from build123d import *

# Parameters (mm, degrees)
EXTRUDE_1_DEPTH     = 0.6
SKETCH_2_W          = 6
SKETCH_2_H          = 0.6
EXTRUDE_2_DEPTH     = 2.5
SKETCH_3_W          = 6
SKETCH_3_H          = 1.9
CUT_EXTRUDE_1_DEPTH = 42.859885332


with BuildPart() as part:
    # 草图1 → 凸台-拉伸1 (new body)
    with BuildSketch(Plane.XY):
        Polygon((0, 0), (11.5, 0), (11.5, 3), (18, 3), (18, 0), (39, 0), (39, 6.8), (33.2, 6.8), (31, 9), (16, 9), (16, 15), (10, 15), (10, 12.5), (0, 12.5), (0, 9), (10, 9), (10, 6.5), (0, 6.5), align=None)
    extrude(amount=EXTRUDE_1_DEPTH)

    # 草图2 → 凸台-拉伸2 (add)
    with BuildSketch(Plane(origin=(0, 0, 0), x_dir=(-1, 0, 0), z_dir=(0, 0, -1))):
        with Locations((-13, 12.8)):
            Rectangle(SKETCH_2_W, SKETCH_2_H)
    extrude(amount=EXTRUDE_2_DEPTH)

    # 草图3 → 切除-拉伸1 (cut, through all)
    with BuildSketch(Plane(origin=(0, 0, 0), x_dir=(-1, 0, 0), z_dir=(0, 0, -1))):
        with Locations((-13, 14.05)):
            Rectangle(SKETCH_3_W, SKETCH_3_H)
    extrude(amount=-CUT_EXTRUDE_1_DEPTH, mode=Mode.SUBTRACT)


solid = part.part
The model under review builds one solid part; all positions refer to its coordinate system, in mm. A direction names the side the tool comes from. Round coordinates to 2 decimals unless told otherwise and drop trailing zeros. Write each loop counter-clockwise with the first axis right and the second up, starting at its lowest first coordinate (ties: lowest second). Pieces come first, ordered by that corner, then holes. Notation, with made-up numbers: M -15.5,-32 L -6.5,-32 A27 cw -6.5,-15 Z; hole C 44.5,-16 d11. An arc over 180 degrees is marked long. Use a Markdown table: item, result. Add a question column.
Q1. To check wall thickness, follow line 1 (Y direction, x = 5, z = 0.25); line 2 (Z direction, x = 4, y = 3.25); line 3 (Y direction, x = 12, z = 0.4). State the ranges of each line that lie inside material, in increasing order.
Q2. We need section C-C, the plane z = -1.4. State the section outline as (x, y) points.
Q3. We need section A-A, the plane x = 15. State the section outline as (y, z) points, plus the area to 3 significant figures.
Q4. Machinability: for faces 1 (the face through (13, 12.5, -1)), 2 (the face through (13, 13.1, -1)), 3 (the face through (16, 11.6, 0.3)), which of the approach directions +Z, -Z, +X, -X, +Y, -Y give a long, thin tool a straight path to every point of the face, cutting with its end or side? Answer none if there is none.
Q5. Insertion check: pin 1 (1.2 mm diameter, centred on x = 11.5, z = -1, fed in from -Y); pin 2 (6 mm diameter, centred on x = 17, y = 4, fed in from -Z); pin 3 (1.5 mm diameter, centred on x = 4.5, y = 8, fed in from +Z); pin 4 (0.5 mm diameter, centred on x = 7, z = 0.5, fed in from +Y). Each pin has a flat end and moves straight along its axis. Give the tip position at first contact, or say it passes through.
Q6. The part is to be moulded in two halves that separate along Z. For faces 4 (the face through (32.1, 7.9, 0.3)), 5 (the face through (19, 5, 0.6)), 6 (the face through (19, 5, 0)), say which applies: pulls with the +Z half, pulls with the -Z half, needs draft (parallel to the pull), parting line crosses it, or undercut.
Q7. We need section B-B, the plane y = 10.75. State the section outline as (x, z) points.
Findings below:
| question | item | result |
|---|---|---|
| 1 | line 1 | y = 0 to 6.5, 9 to 12.5 |
| 1 | line 2 | z = 0 to 0.6 |
| 1 | line 3 | y = 3 to 13.1 |
| 2 | outline | M 10,12.5 L 16,12.5 L 16,13.1 L 10,13.1 Z |
| 3 | outline | M 3,0 L 12.5,0 L 12.5,-2.5 L 13.1,-2.5 L 13.1,0.6 L 3,0.6 Z |
| 3 | area | 7.56 mm² |
| 4 | face 1 | -Z, +X, -X, -Y |
| 4 | face 2 | +Z, -Z, +X, -X, +Y |
| 4 | face 3 | +Z, -Z, +X, +Y |
| 5 | pin 1 | stops at y = 12.5 |
| 5 | pin 2 | stops at z = 0 |
| 5 | pin 3 | passes through |
| 5 | pin 4 | stops at y = 12.5 |
| 6 | face 4 | needs draft |
| 6 | face 5 | pulls with the +Z half |
| 6 | face 6 | pulls with the -Z half |
| 7 | outline | M 0,0 L 16,0 L 16,0.6 L 0,0.6 Z |
